Geometry check sheet. Reference: the model listing, model coordinates, mm. Face numbers are marked on the shaded views. Coordinates: 2 decimals unless noted, no trailing zeros. Loops run counter-clockwise (first coordinate to the right, second up) from the corner with the lowest first, then second, coordinate; pieces in that order, holes last.
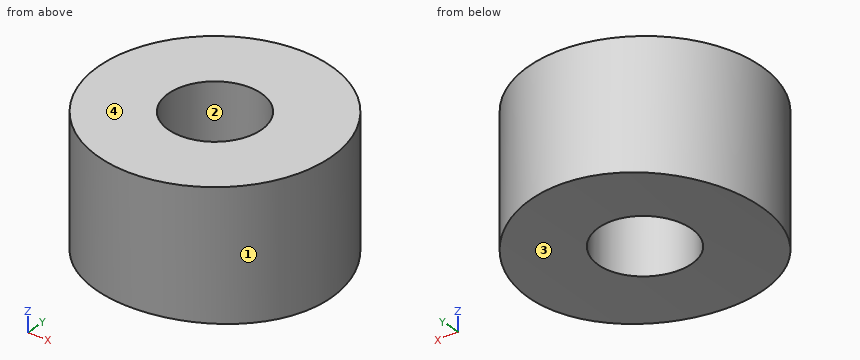
from build123d import *

# Parameters (mm, degrees)
CYLINDER003_R          = 48
CYLINDER003_DEPTH      = 245
CYLINDER003_ROLL_ANGLE = 90
CYLINDER001_R          = 2
CYLINDER001_DEPTH      = 6.4
CYLINDER_R             = 5
CYLINDER_DEPTH         = 6.4


with BuildPart() as cilindro:
    # Cylinder003 → Cylinder003 (new body)
    with BuildSketch(Plane.XY):
        Circle(CYLINDER003_R)
    extrude(amount=CYLINDER003_DEPTH)


with BuildPart() as cilindro_1:
    # Cylinder003 roll: moved
    add(cilindro.part.rotate(Axis((0, 0, 0), (1, 0, 0)), CYLINDER003_ROLL_ANGLE))


with BuildPart() as cilindro_2:
    # Cylinder003 placement: moved
    add(cilindro_1.part.moved(Location((0, 79, -47))))


with BuildPart() as bumper_taladro:
    # Cylinder001 → Cylinder001 (new body)
    with BuildSketch(Plane.XY):
        Circle(CYLINDER001_R)
    extrude(amount=CYLINDER001_DEPTH)


with BuildPart() as bumper_para_m2_temporal:
    # Cylinder → Cylinder (new body)
    with BuildSketch(Plane.XY):
        Circle(CYLINDER_R)
    extrude(amount=CYLINDER_DEPTH)

    # Cut: cut Bumper taladro
    add(bumper_taladro.part, mode=Mode.SUBTRACT)

    # Cut001: cut Cilindro
    add(cilindro_2.part, mode=Mode.SUBTRACT)


solid = bumper_para_m2_temporal.part
1) Material ranges on probe 1 along X at (y, z) = (0, 4.75); probe 2 along Z at (x, y) = (2, -0.5), recorded low to high.
Data:
probe 1: x = -5 to -2, 2 to 5
probe 2: z = 0.96 to 6.4
2) Section check A-A on x = 0. Record the cut outline in (y, z).
Data:
outline: (-5, 1) - (-2, 1) - (-2, 6.4) - (-5, 6.4) - close; (2, 1) - (5, 1) - (5, 6.4) - (2, 6.4) - close
3) Mould release check, pull along X, two halves, no side actions. Record for the marked faces 1, 2, 3 and 4: +X half, -X half, draft (parallel to the pull), parting line (faces both ways), or undercut.
Data:
face 1: parting line
face 2: undercut
face 3: undercut
face 4: draft
4) Section check B-B on y = 0. Record the cut outline in (x, z), and give its area (3 significant figures).
Data:
outline: (-5, 0.74) arc R48 cw to (-2, 0.96) - (-2, 6.4) - (-5, 6.4) - close; (2, 0.96) arc R48 cw to (5, 0.74) - (5, 6.4) - (2, 6.4) - close
area: 33.2 mm2
5) Section check D-D on y = 2.25. Record the cut outline in (x, z), and give its area (3 significant figures).
Data:
outline: (-4.47, 0.79) arc R48 cw to (4.47, 0.79) - (4.47, 6.4) - (-4.47, 6.4) - close
area: 48.8 mm2
6) Section check C-C on z = 5.05. Record the cut outline in (x, y).
Data:
outline: circle Ø10 at (0, 0); hole circle Ø4 at (0, 0)
7) Depth check by flat-ended pin: pin 1 (3 mm diameter, centred on y = -4, z = 5.5, fed in from +X); pin 2 (1 mm diameter, centred on x = 2.5, z = 4, fed in from +Y); pin 3 (1 mm diameter, centred on x = -3.5, z = 5.5, fed in from -Y). Enter the tip coordinate at first touch or a pass-through.
Data:
pin 1: stops at x = 4.33
pin 2: stops at y = 4.58
pin 3: stops at y = -4
